Autodesk Inventor part; units mm, degrees
ref_plane "YZ Plane" through (0, 0, 0) normal (1, 0, 0) x (0, 1, 0)
ref_plane "XZ Plane" through (0, 0, 0) normal (0, 1, 0) x (-1, 0, 0)
ref_plane "XY Plane" through (0, 0, 0) normal (0, 0, 1) x (1, 0, 0)
sketch "block" plane through (0, 0, 0) normal (0, 1, 0) x (-1, 0, 0)
  line L0 (0, 0) -> (-200, 0)
  line L1 (-200, 0) -> (-200, -250)
  line L2 (-200, -250) -> (0, -250)
  line L3 (0, -250) -> (0, 0)
  dimension "d31" = 200
  dimension "d32" = 250
extrude "ext_block" add sketch "block" against normal blind 24
shell "Shell2" thickness 3 removed faces 0
sketch "lines_base" plane through (0, 0, 0) normal (0, 1, 0) x (-1, 0, 0)
  line L0 (0, 0) -> (-200, 0)
  line L1 (-200, 0) -> (-200, -250)
  line L2 (-200, -250) -> (0, -250)
  line L3 (0, -250) -> (0, 0)
  circle A0 centre (-65, -60) radius 6
  circle A1 centre (-125, -80) radius 6
  circle A2 centre (-65, -60) radius 12.5
  circle A3 centre (-65, -60) radius 8.5
  circle A4 centre (-125, -80) radius 8.5
  circle A5 centre (-125, -80) radius 12.5
  circle A6 centre (-175, -125) radius 3
  line L4 (-175, -125) -> (-175, -209)
  line L5 (-175, -125) -> (-91, -125) construction
  circle A7 centre (-175, -139) radius 3
  circle A8 centre (-175, -153) radius 3
  circle A9 centre (-175, -167) radius 3
  circle A10 centre (-175, -181) radius 3
  circle A11 centre (-175, -195) radius 3
  circle A12 centre (-175, -209) radius 3
  circle A13 centre (-95, -185) radius 2.5
  circle A14 centre (-95, -185) radius 5
  point P0 (-200, -125)
  dimension "d0" = 200
  dimension "d1" = 250
  dimension "d2" = 12
  dimension "d3" = 12
  dimension "d4" = 25
  dimension "d5" = 17
  dimension "d6" = 17
  dimension "d7" = 25
  dimension "d8" = 75
  dimension "d9" = 80
  dimension "d10" = 65
  dimension "d11" = 60
  dimension "d12" = 6
  dimension "d13" = 84
  dimension "d14" = 90
  dimension "d15" = 25
  dimension "d16" = 125
  dimension "d19" = 14
  dimension "d24" = 5
  dimension "d25" = 10
  dimension "d26" = 65
  dimension "d27" = 95
extrude "holes" cut sketch "lines_base" against normal up to surface (3 mm away) contours A0 | A1 | A6 | A7 L4 | L4 A7 | A8 L4 | L4 A8 | A9 L4 | L4 A9 | A10 L4 | L4 A10 | A11 L4 | L4 A11 | A12 | A13
sketch "Sketch4" plane through (200, 0, -250) normal (0, 0, -1) x (-1, 0, 0)
  line L0 (188, -4) -> (169, -4)
  line L1 (169, -4) -> (169, -17)
  line L2 (169, -17) -> (188, -17)
  line L3 (188, -17) -> (188, -4)
  line L4 (0, 0) -> (200, 0)
  line L5 (200, 0) -> (200, -24)
  dimension "d40" = 19
  dimension "d41" = 13
  dimension "d42" = 4
  dimension "d43" = 12
extrude "pwr_button_hole" cut sketch "Sketch4" against normal up to surface (3 mm away)
ref_plane "Work Plane1" through (7, -21, -243) normal (0, 1, 0) x (1, 0, 0)
sketch "Sketch5" plane through (7, -21, -243) normal (0, 1, 0) x (1, 0, 0)
  line L0 (-20.9366, 21.7948) -> (229.9216, 21.7948)
  line L1 (229.9216, 21.7948) -> (229.9216, -260.9184)
  line L2 (229.9216, -260.9184) -> (-20.9366, -260.9184)
  line L3 (-20.9366, -260.9184) -> (-20.9366, 21.7948)
  point P0 (-7, -243)
extrude "back_cover_cut" cut sketch "Sketch5" against normal through all
sketch "Sketch10" plane through (3, -3, -3) normal (0, -1, 0) x (1, 0, 0)
  line L0 (213.1188, 33.5044) -> (-22.0421, 33.5044)
  line L1 (-22.0421, 33.5044) -> (-22.0421, -278.1947)
  line L2 (-22.0421, -278.1947) -> (213.1188, -278.1947)
  line L3 (213.1188, -278.1947) -> (213.1188, 33.5044)
  point P0 (-3, 3)
extrude "Extrusion8" cut sketch "Sketch10" along normal through all
properties part number "back_top" material "Glass"
Read the model definition and answer for the solid it produces. Units are mm, in the model's axes. Round coordinates to 2 decimals unless told otherwise and drop trailing zeros. Write each loop counter-clockwise with the first axis right and the second up, starting at its lowest first coordinate (ties: lowest second). Pieces come first, ordered by that corner, then holes. Notation, with made-up numbers: M 74.5,51.5 L 99.5,51.5 A17 ccw 99.5,84.5 Z; hole C 84,42 d3. An arc over 180 degrees is marked long. Use a Markdown table: item, result.
1) The part is cut by section A-A (z = -60). Write down the section's boundary in (x, y), plus the area to 3 significant figures.
Answers follow:
| item | result |
|---|---|
| outline | M 0,-3 L 59,-3 L 59,0 L 0,0 Z; M 71,-3 L 200,-3 L 200,0 L 71,0 Z |
| area | 564 mm2 |
2) The part is cut by section B-B (x = 175). Give the number of separate pieces and of enclosed holes in the cut face, plus the area to 3 significant figures.
Answers follow:
| item | result |
|---|---|
| separate pieces | 8 |
| enclosed holes | 0 |
| area | 624 mm2 |
3) For a pull along Z with two mould halves and no side action, classify faces 1 (the flat face through (101, 0, -123)), 2 (the cylindrical face through (71, -1, -60)) as pulls with the +Z half, pulls with the -Z half, needs draft (parallel to the pull), parting line crosses it, or undercut.
Answers follow:
| item | result |
|---|---|
| face 1 | needs draft |
| face 2 | undercut |
4) The part is cut by section C-C (x = 125). Write down the section's boundary in (y, z), plus the area to 3 significant figures.
Answers follow:
| item | result |
|---|---|
| outline | M -3,-250 L 0,-250 L 0,-86 L -3,-86 Z; M -3,-74 L 0,-74 L 0,0 L -3,0 Z |
| area | 714 mm2 |
5) Straight lines are drawn through the part: line 1 along X through (y, z) = (-2.8, -180.5); line 2 along Z through (x, y) = (125, -1.9); line 3 along Z through (x, y) = (65, -1.35). For each, find the intervals that lie inside material, in ascending order. Write a range as [from, to].
Answers follow:
| item | result |
|---|---|
| line 1 | x = [0, 172.04], [177.96, 200] |
| line 2 | z = [-250, -86], [-74, 0] |
| line 3 | z = [-250, -66], [-54, 0] |
